For this review, take the finished solid that the model builds, in its own axes (mm). A direction names the side the tool comes from. Give positions to 0.01 mm unless a question says otherwise; leave off trailing zeros. Loops run counter-clockwise (first coordinate to the right, second up) from the corner with the lowest first, then second, coordinate; pieces in that order, holes last. Notation, with made-up numbers: (-12, -38.75) - (35, -38.75) arc R38 cw to (35, 0.25) - close; hole circle Ø11 at (74.25, 71.5). An arc over 180 degrees is marked (long way). Put each result on its own line as item: value. Start each with the question number.
from build123d import *

# Parameters (mm, degrees)
SKETCH1_R           = 5
BOSS_EXTRUDE1_DEPTH = 19
SKETCH2_R           = 6
BOSS_EXTRUDE2_DEPTH = 3
SKETCH3_R           = 5
BOSS_EXTRUDE3_DEPTH = 3
SKETCH4_R           = 2
BOSS_EXTRUDE4_DEPTH = 107
SKETCH5_RX          = 10
SKETCH5_RY          = 7.5
BOSS_EXTRUDE5_DEPTH = 4
SKETCH6_R           = 2
BOSS_EXTRUDE6_DEPTH = 4
FILLET1_R           = 1
SKETCH7_R           = 2.5
CUT_EXTRUDE1_DEPTH  = 11


with BuildPart() as part:
    # Sketch1 → Boss-Extrude1 (new body)
    with BuildSketch(Plane.XY):
        Circle(SKETCH1_R)
    extrude(amount=BOSS_EXTRUDE1_DEPTH)

    # Sketch2 → Boss-Extrude2 (add)
    with BuildSketch(Plane(origin=(0, 0, 0), x_dir=(-1, 0, 0), z_dir=(0, 0, -1))):
        Circle(SKETCH2_R)
    extrude(amount=BOSS_EXTRUDE2_DEPTH)

    # Sketch3 → Boss-Extrude3 (add)
    with BuildSketch(Plane(origin=(0, 0, -3), x_dir=(-1, 0, 0), z_dir=(0, 0, -1))):
        Circle(SKETCH3_R)
    extrude(amount=BOSS_EXTRUDE3_DEPTH)

    # Sketch4 → Boss-Extrude4 (add)
    with BuildSketch(Plane(origin=(0, 0, -6), x_dir=(-1, 0, 0), z_dir=(0, 0, -1))):
        Circle(SKETCH4_R)
    extrude(amount=BOSS_EXTRUDE4_DEPTH)



with BuildPart() as body_2:
    # Sketch5 → Boss-Extrude5 (new body, symmetric)
    with BuildSketch(Plane(origin=(0, 0, 0), x_dir=(0, 0, -1), z_dir=(1, 0, 0))):
        with Locations(Location((-31.48355656, 0), (0, 0, 180))):
            Ellipse(SKETCH5_RX, SKETCH5_RY)
    extrude(amount=BOSS_EXTRUDE5_DEPTH, both=True)


with BuildPart() as part_1:
    add(part.part)

    add(body_2.part)  # Boss-Extrude6 merges body 2
    # Sketch6 → Boss-Extrude6 (add)
    with BuildSketch(Plane.XY.offset(19)):
        Circle(SKETCH6_R)
    extrude(amount=BOSS_EXTRUDE6_DEPTH)

    # Fillet1
    fillet1_edges = [part_1.edges().sort_by_distance(p)[0] for p in [
        (-4, 0.002625288, 21.483557173),
        (4, 0.002625288, 21.483557173),
    ]]
    fillet(fillet1_edges, radius=FILLET1_R)

    # Sketch7 → Cut-Extrude1 (cut, through all)
    with BuildSketch(Plane(origin=(4, 0, 0), x_dir=(0, 0, -1), z_dir=(1, 0, 0))):
        with Locations((-31.444890306, 0)):
            Circle(SKETCH7_R)
    extrude(amount=-CUT_EXTRUDE1_DEPTH, mode=Mode.SUBTRACT)


solid = part_1.part
1) Machinability: for faces 1 (the flat face through (-4, 2, 29)), 2 (the flat face through (-0.1, -2.2, 19)), 3 (the flat face through (0, 0, -113)), 4 (the cylindrical face through (0, -2, -59)), 5 (the flat face through (4, 2, 29)), which of the approach directions +Z, -Z, +X, -X, +Y, -Y give a long, thin tool a straight path to every point of the face, cutting with its end or side? Answer none if there is none.
2) Insertion check: P1, Ø6.5, axis at y = 0.5, z = 29.5, coming from the -X side; P2, Ø4, axis at y = -2, z = 34, coming from the +X side; P3, Ø3.5, axis at x = 1.5, y = -2.5, coming from the +Z side. Each pin has a flat end and moves straight along its axis. Give the tip position at first contact, or say it passes through.
3) Wall thickness on probe 1 along Z at (x, y) = (4.5, -1.75); probe 2 along Y at (x, z) = (0, -12); probe 3 along X at (y, z) = (5.25, 26): over which ranges is each line inside the solid? List them lowest first.
4) Take a section at A-A on z = -38. State the section outline as (x, y) points.
5) Take a section at B-B on z = 11. State the section outline as (x, y) points.
6) Mouldability with a two-part tool opening along Z and no side actions: class faces 6 (the flat face through (4, 4, -3)), 7 (the flat face through (4, 4, 0)), 8 (the cylindrical face through (-1.08, -4.88, 9.37)), 9 (the cylindrical face through (1.08, -4.88, -4.48)) as released by +Z, released by -Z, zero draft, split by the parting line, or undercut.
Answers follow:
1. face 1: +Z, -X, +Y, -Y
1. face 2: none
1. face 3: -Z, +X, -X, +Y, -Y
1. face 4: -Z
1. face 5: +Z, +X, +Y, -Y
2. P1: x = -4
2. P2: x = 4
2. P3: z = 41.43
3. probe 1: -6 to 19
3. probe 2: -2 to 2
3. probe 3: -4 to 4
4. outline: circle Ø4 at (0, 0)
5. outline: circle Ø10 at (0, 0)
6. face 6: released by -Z
6. face 7: undercut
6. face 8: undercut
6. face 9: zero draft
